The drawing under review shows one solid part. Ordinate dimensions are in mm from its lowest x, y, z. A direction names the side the tool comes from. Give positions to 0.01 mm unless a question says otherwise; leave off trailing zeros. Write each loop counter-clockwise with the first axis right and the second up, starting at its lowest first coordinate (ties: lowest second). Pieces come first, ordered by that corner, then holes. Notation, with made-up numbers: (-6, 10) - (43, 10) arc R18 ccw to (43, 37) - close; hole circle Ø10 at (10.25, -32.5). An arc over 180 degrees is marked (long way). Write each question's results on one line, items separated by ' | '. Start each with the question number.
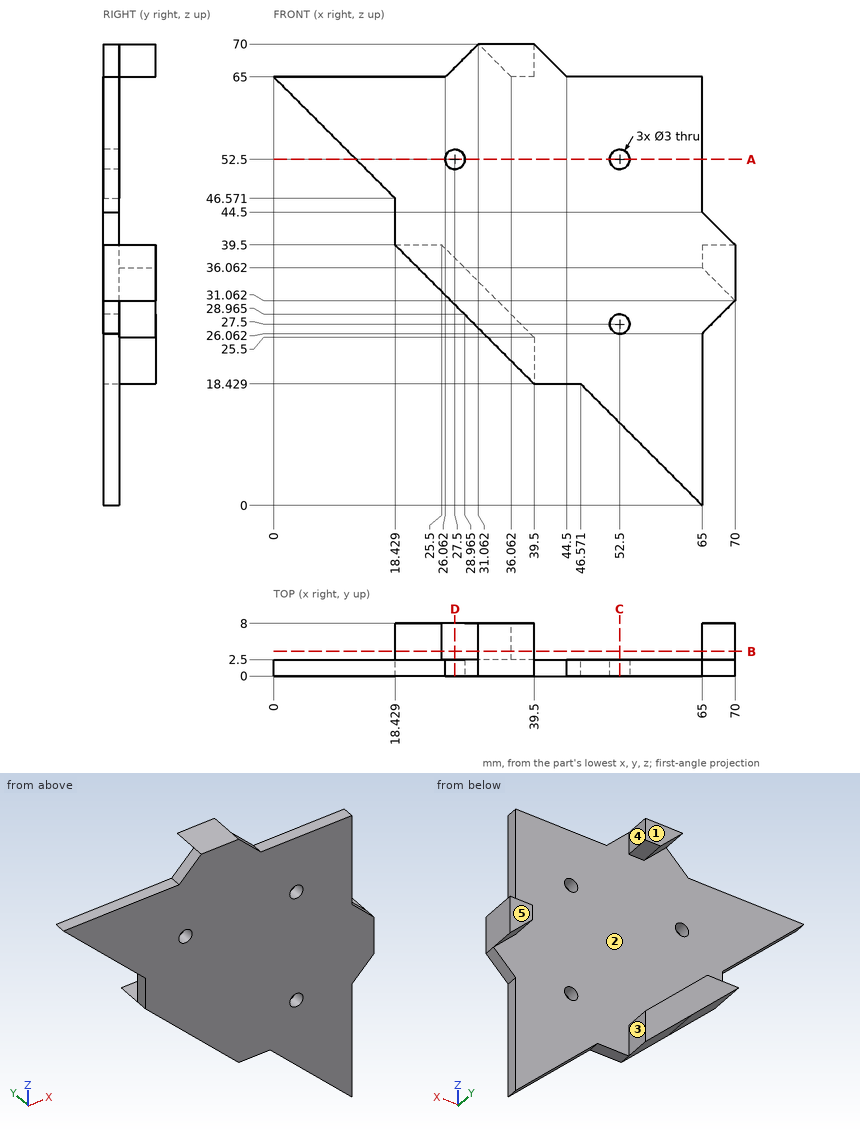
Q1. Add section C-C on x = 52.5. State the section outline as (y, z) points.
Q2. Insertion check: P1, Ø4, axis at y = 6, z = 67, coming from the +X side; P2, Ø3, axis at y = 1.5, z = 41.5, coming from the -X side; P3, Ø2, axis at y = 1, z = 37, coming from the -X side. Each pin has a flat end and moves straight along its axis. Give the tip position at first contact, or say it passes through.
Q3. For line 1 along Z through (x, y) = (52.5, 1.7); line 2 along Y through (x, z) = (11, 59.5), list the stretches that pass through material, from the lowest coordinate up. Write a range as [from, to].
Q4. Add section A-A on z = 52.5. State the section outline as (x, y) points, plus the area to 3 significant figures.
Q5. Add section B-B on y = 3.75. State the section outline as (x, z) points (1 decimal).
Q6. The part is to be moulded in two halves that separate along X. For the marked faces 1, 2 and 3, say which applies: +X half, -X half, draft (parallel to the pull), parting line (faces both ways), or undercut.
Q7. Machinability: for the marked faces 4 and 5, which of the approach directions +Z, -Z, +X, -X, +Y, -Y give a long, thin tool a straight path to every point of the face, cutting with its end or side? Answer none if there is none.
Q8. Add section D-D on x = 27.5. State the section outline as (y, z) points.
Result:
1) outline: (0, 12.5) - (2.5, 12.5) - (2.5, 26) - (0, 26) - close; (0, 29) - (2.5, 29) - (2.5, 51) - (0, 51) - close; (0, 54) - (2.5, 54) - (2.5, 65) - (0, 65) - close
2) P1: stops at x = 39.5 | P2: stops at x = 18.43 | P3: stops at x = 19.93
3) line 1: z = [12.5, 26], [29, 51], [54, 65] | line 2: y = [0, 2.5]
4) outline: (12.5, 0) - (26, 0) - (26, 2.5) - (12.5, 2.5) - close; (29, 0) - (51, 0) - (51, 2.5) - (29, 2.5) - close; (54, 0) - (65, 0) - (65, 2.5) - (54, 2.5) - close | area: 116 mm²
5) outline: (18.4, 39.5) - (29, 29) - (39.5, 18.4) - (39.5, 25.5) - (25.5, 39.5) - close; (31.1, 70) - (36.1, 65) - (39.5, 65) - (39.5, 70) - close; (65, 36.1) - (70, 31.1) - (70, 39.5) - (65, 39.5) - close
6) face 1: draft | face 2: undercut | face 3: +X half
7) face 4: +Z, -Z, +X, +Y | face 5: +Z, -Z, +X, -X, +Y
8) outline: (0, 30.43) - (8, 30.43) - (8, 37.5) - (2.5, 37.5) - (2.5, 51) - (0, 51) - close; (0, 54) - (2.5, 54) - (2.5, 66.44) - (0, 66.44) - close
